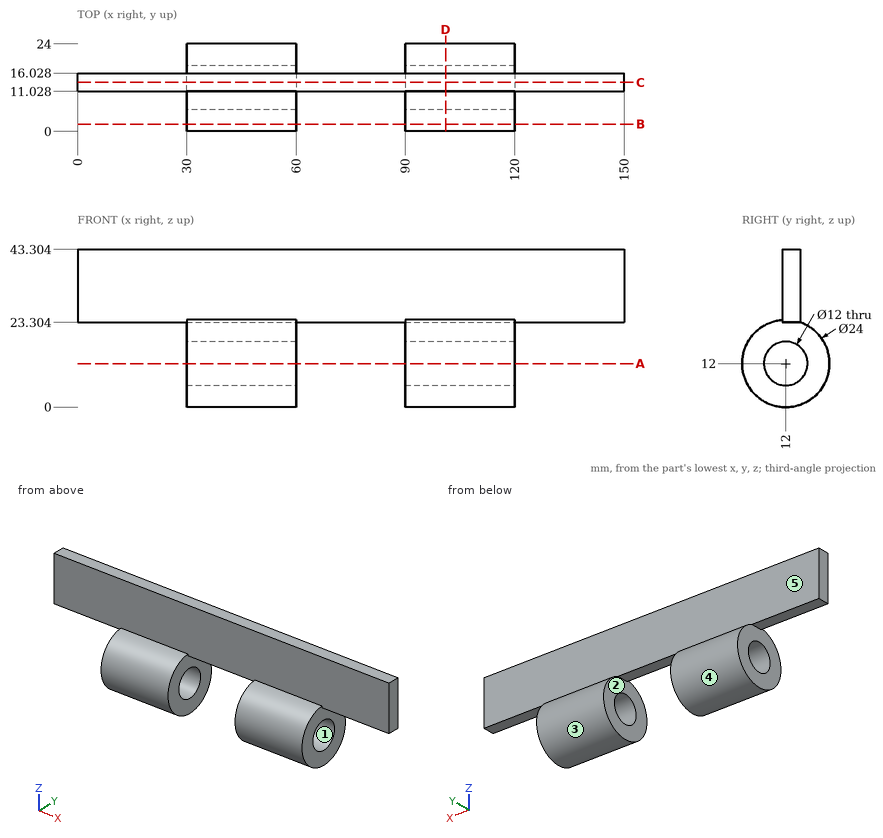
For this review, use the dimensioned drawing (mm, ordinates from the lowest corner) and the shaded views. A direction names the side the tool comes from. Round coordinates to 2 decimals unless told otherwise and drop trailing zeros. Order: outer loops, then holes, each group sorted by start corner. A loop starts at its lowest first (then second) coordinate and runs counter-clockwise, first axis right, second up.
1) Draft analysis for pull direction Z (two halves, no side actions). For the marked faces 1, 2 and 3, state which applies: released by +Z, released by -Z, zero draft, split by the parting line, or undercut.
The answers:
face 1: undercut
face 2: zero draft
face 3: split by the parting line
2) For L1, parallel to Y at x = 107.5, z = 12; L2, parallel to X at y = 17.25, z = 7; L3, parallel to Z at x = 76, y = 12, list the stretches that pass through material, from the lowest coordinate up.
The answers:
L1: y = 0 to 6, 18 to 24
L2: x = 30 to 60, 90 to 120
L3: z = 23.3 to 43.3
3) Consider section C-C (y = 13.5). State the section outline as (x, z) points (1 decimal).
The answers:
outline: (0, 23.3) - (30, 23.3) - (30, 17.8) - (60, 17.8) - (60, 23.3) - (90, 23.3) - (90, 17.8) - (120, 17.8) - (120, 23.3) - (150, 23.3) - (150, 43.3) - (0, 43.3) - close; (30, 0.1) - (60, 0.1) - (60, 6.2) - (30, 6.2) - close; (90, 0.1) - (120, 0.1) - (120, 6.2) - (90, 6.2) - close
4) Machinability: for the marked faces 4 and 5, which of the approach directions +Z, -Z, +X, -X, +Y, -Y give a long, thin tool a straight path to every point of the face, cutting with its end or side? Answer none if there is none.
The answers:
face 4: +X, -X
face 5: +Z, +X, -X, +Y
5) Consider section D-D (x = 101). State the section outline as (y, z) points, plus the area to 3 significant figures.
The answers:
outline: (11.03, 23.96) arc R12 ccw (long way) to (16.03, 23.3) - (16.03, 43.3) - (11.03, 43.3) - close; hole circle Ø12 at (12, 12)
area: 437 mm2
6) Clearance check with flat-ended pins moving along their axes: pin 1 Ø4 at (x, y) = (132.5, 13.5) entering from -Z; pin 2 Ø7 at (y, z) = (13.5, 7) entering from +X; pin 3 Ø16 at (x, z) = (51.5, 32.5) entering from +Y. State where each tip first meets the part, or that it passes through.
The answers:
pin 1: stops at z = 23.3
pin 2: stops at x = 120
pin 3: stops at y = 16.03
7) Consider section B-B (y = 2). State the section outline as (x, z) points.
The answers:
outline: (30, 5.37) - (60, 5.37) - (60, 18.63) - (30, 18.63) - close; (90, 5.37) - (120, 5.37) - (120, 18.63) - (90, 18.63) - close
8) Consider section A-A (z = 12). State the section outline as (x, y) points.
The answers:
outline: (30, 0) - (60, 0) - (60, 6) - (30, 6) - close; (30, 18) - (60, 18) - (60, 24) - (30, 24) - close; (90, 0) - (120, 0) - (120, 6) - (90, 6) - close; (90, 18) - (120, 18) - (120, 24) - (90, 24) - close
